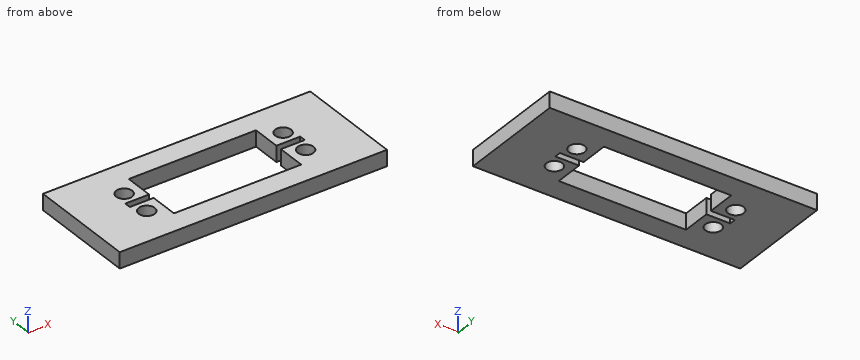
Autodesk Inventor part; units mm, degrees
ref_plane "YZ Plane" through (0, 0, 0) normal (1, 0, 0) x (0, 1, 0)
ref_plane "XZ Plane" through (0, 0, 0) normal (0, 1, 0) x (-1, 0, 0)
ref_plane "XY Plane" through (0, 0, 0) normal (0, 0, 1) x (1, 0, 0)
sketch "Sketch1" plane through (0, 0, 0) normal (0, 0, 1) x (1, 0, 0)
  line L0 (-26, 13) -> (26, 13)
  line L1 (26, -13) -> (-26, -13)
  line L2 (-26, 13) -> (26, -13) construction
  line L3 (26, 13) -> (-26, -13) construction
  line L4 (-54.6, 22.1) -> (54.6, 22.1)
  line L5 (54.6, 22.1) -> (54.6, -22.1)
  line L6 (54.6, -22.1) -> (-54.6, -22.1)
  line L7 (-54.6, -22.1) -> (-54.6, 22.1)
  line L8 (-54.6, 22.1) -> (54.6, -22.1) construction
  line L9 (54.6, 22.1) -> (-54.6, -22.1) construction
  line L10 (-26, 1.3) -> (-35.75, 1.3)
  line L11 (-35.75, 1.3) -> (-35.75, -1.3)
  line L12 (-35.75, -1.3) -> (-26, -1.3)
  line L13 (26, 1.3) -> (35.75, 1.3)
  line L14 (35.75, 1.3) -> (35.75, -1.3)
  line L15 (35.75, -1.3) -> (26, -1.3)
  line L16 (-26, 1.3) -> (-26, 13)
  line L17 (-26, -13) -> (-26, -1.3)
  line L18 (26, -1.3) -> (26, -13)
  line L19 (26, 1.3) -> (26, 13)
  point P0 (0, 0)
  point P1 (-35.75, 0)
  point P2 (0, 0)
  dimension "CInt" = 52
  dimension "LInt" = 26
  dimension "Cext" = 109.2
  dimension "Lext" = 44.2
  dimension "Cpeq" = 9.75
  dimension "Lpeq" = 2.6
  dimension "d10" = 9.75
  dimension "d11" = 2.6
extrude "Extrusion1" add sketch "Sketch1" along normal mid plane 6.5
sketch "Sketch8" plane through (0, 0, 3.25) normal (0, 0, 1) x (1, 0, 0)
  point P0 (0, 0)
hole "Hole1" at (-32.5, 6.5, 3.25) direction (0, 0, -1) diameter 6.5 end through all
pattern_linear "Rectangular Pattern1" count 2 spacing 13 along (0, -1, 0) of "Hole1"
hole "Hole2" at (32.5, 6.6, 3.25) direction (0, 0, -1) diameter 6.5 end through all
pattern_linear "Rectangular Pattern2" count 2 spacing 13 along (0, -1, 0) of "Hole2"
properties part number "Cou-3"
Geometry: final body of the model. Coordinates: model frame, mm. Give positions to 0.01 mm unless a question says otherwise; leave off trailing zeros. Write each loop counter-clockwise with the first axis right and the second up, starting at its lowest first coordinate (ties: lowest second). Pieces come first, ordered by that corner, then holes. Notation, with made-up numbers: (52, -11.75) - (72, -11.75) arc R15 ccw to (72, 1.25) - close; hole circle Ø6 at (12, -16.75). An arc over 180 degrees is marked (long way). Return JSON: item names as keys, results as strings. Group by question number.
1) Line query: line 1 (X direction, y = 6.6, z = 0); line 2 (Y direction, x = 32.5, z = 1.25); line 3 (Y direction, x = -32.5, z = 1). Output: solid intervals per line, ascending.
2) First-contact query: P1, Ø6, axis at x = 32.5, y = 6.6, coming from the +Z side. Flat tip, straight axial feed; report the tip coordinate or a pass-through.
3) Section B-B on y = 0. Return the cut outline in (x, z).
4) Section C-C on z = -2. Return the cut outline in (x, y).
5) Section A-A on x = 32.5. Return the cut outline in (y, z), plus the area to 3 significant figures.
6) Section D-D on y = -6.5. Return the cut outline in (x, z).
Filled in:
{
 "1": {"line 1": "x = -54.6 to -35.75, -29.25 to -26, 26 to 29.25, 35.75 to 54.6", "line 2": "y = -22.1 to -9.65, -3.15 to -1.3, 1.3 to 3.35, 9.85 to 22.1", "line 3": "y = -22.1 to -9.75, -3.25 to -1.3, 1.3 to 3.25, 9.75 to 22.1"},
 "2": {"P1": "passes through"},
 "3": {"outline": "(-54.6, -3.25) - (-35.75, -3.25) - (-35.75, 3.25) - (-54.6, 3.25) - close; (35.75, -3.25) - (54.6, -3.25) - (54.6, 3.25) - (35.75, 3.25) - close"},
 "4": {"outline": "(-54.6, -22.1) - (54.6, -22.1) - (54.6, 22.1) - (-54.6, 22.1) - close; hole circle Ø6.5 at (-32.5, -6.5); hole (-35.75, -1.3) - (-26, -1.3) - (-26, -13) - (26, -13) - (26, -1.3) - (35.75, -1.3) - (35.75, 1.3) - (26, 1.3) - (26, 13) - (-26, 13) - (-26, 1.3) - (-35.75, 1.3) - close; hole circle Ø6.5 at (-32.5, 6.5); hole circle Ø6.5 at (32.5, -6.4); hole circle Ø6.5 at (32.5, 6.6)"},
 "5": {"outline": "(-22.1, -3.25) - (-9.65, -3.25) - (-9.65, 3.25) - (-22.1, 3.25) - close; (-3.15, -3.25) - (-1.3, -3.25) - (-1.3, 3.25) - (-3.15, 3.25) - close; (1.3, -3.25) - (3.35, -3.25) - (3.35, 3.25) - (1.3, 3.25) - close; (9.85, -3.25) - (22.1, -3.25) - (22.1, 3.25) - (9.85, 3.25) - close", "area": "186 mm^2"},
 "6": {"outline": "(-54.6, -3.25) - (-35.75, -3.25) - (-35.75, 3.25) - (-54.6, 3.25) - close; (-29.25, -3.25) - (-26, -3.25) - (-26, 3.25) - (-29.25, 3.25) - close; (26, -3.25) - (29.25, -3.25) - (29.25, 3.25) - (26, 3.25) - close; (35.75, -3.25) - (54.6, -3.25) - (54.6, 3.25) - (35.75, 3.25) - close"}
}
